The model under review builds one solid part; all positions refer to its coordinate system, in mm. A direction names the side the tool comes from. Coordinates: 2 decimals unless noted, no trailing zeros. One line per item, written item: value.
```python
from build123d import *

# Parameters (mm, degrees)
SKETCH3_R           = 3.512937447
SKETCH3_R_2         = 2.5
BOSS_EXTRUDE3_DEPTH = 13
CUT_EXTRUDE9_START  = -13.999999262
CUT_EXTRUDE9_DEPTH  = 13.999999262


# Read off the part's stored shape, not the designer's step: Cut-Extrude9
with BuildPart() as part:
    # Sketch1 → Revolve1 (revolve)
    with BuildSketch(Plane.XY, mode=Mode.PRIVATE) as revolve1_sk:
        with BuildLine():
            Line((-5.977318778, 9), (5.977318778, 9))
            add(Edge.make_bspline(
                [(5.977318778, 9), (5.971811367, 8.975222227), (5.562087836, 7.215033632), (4.069266539, 5.252557202), (1.935066771, 3.855081597), (0.019003444, 3.516133425), (0, 3.512937447)],
                knots=[0.019778015, 0.019778015, 0.019778015, 0.024722519, 0.375, 0.625, 0.982243258, 0.985794607, 0.985794607, 0.985794607], degree=2))
            Line((0, 3.512937447), (0, 2.5))
            add(Edge.make_bspline(
                [(6.999999581, 9.002422396), (5.87124706, 3.409561407), (0, 2.5)],
                knots=[0, 0, 0, 1, 1, 1], degree=2))
            Line((6.999999581, 9.002422396), (6.999999581, 11.002422396))
            Line((6.999999581, 11.002422396), (5.999999581, 11.002422396))
            Line((5.999999581, 11.002422396), (5.999999581, 10.9))
            ThreePointArc((5.999999581, 10.9), (5.736395684, 10.263603897), (5.099999581, 10))
            Line((5.099999581, 10), (-5.099999581, 10))
            ThreePointArc((-5.099999581, 10), (-5.736395684, 10.263603897), (-5.999999581, 10.9))
            Line((-5.999999581, 10.9), (-5.999999581, 11.002422396))
            Line((-5.999999581, 11.002422396), (-6.999999581, 11.002422396))
            Line((-6.999999581, 11.002422396), (-6.999999581, 9.002422396))
            Line((-6.999999581, 9.002422396), (-5.977318778, 9))
        make_face()
    revolve(revolve1_sk.sketch.rotate(Axis((0, 0, 0), (1, 0, 0)), 90), axis=Axis((0, 0, 0), (1, 0, 0)))

    # Sketch3 → Boss-Extrude3 (add)
    with BuildSketch(Plane.ZY.offset(6.999999581)):
        Circle(SKETCH3_R)
        Circle(SKETCH3_R_2, mode=Mode.SUBTRACT)
    extrude(amount=-BOSS_EXTRUDE3_DEPTH)

    # Cut-Extrude9 outline → Cut-Extrude9 (cut)
    with BuildSketch(Plane(origin=(6.999999581, 0, 0), x_dir=(0, 0, -1), z_dir=(1, 0, 0)).offset(CUT_EXTRUDE9_START)):
        with BuildLine():
            ThreePointArc((2.343182528, 2.617293478), (2.746525092, 2.190280673), (3.07307963, 1.702031461))
            Line((3.07307963, 1.702031461), (7.875221607, 4.361707651))
            ThreePointArc((7.875221607, 4.361707651), (7.038377248, 5.612918556), (6.004752201, 6.707202099))
            Line((6.004752201, 6.707202099), (2.343182528, 2.617293478))
        make_face()
        with BuildLine():
            ThreePointArc((3.50723285, -0.200118078), (3.424860771, -0.781702122), (3.24673559, -1.341431145))
            Line((3.24673559, -1.341431145), (8.320240718, -3.437615944))
            ThreePointArc((8.320240718, -3.437615944), (8.776712871, -2.003227439), (8.98780352, -0.512832208))
            Line((8.98780352, -0.512832208), (3.50723285, -0.200118078))
        make_face()
        with BuildLine():
            ThreePointArc((-0.585332029, 3.463829661), (0, 3.512937447), (0.585332029, 3.463829661))
            Line((0.585332029, 3.463829661), (1.5, 8.876576423))
            ThreePointArc((1.5, 8.876576423), (0, 9.002422396), (-1.5, 8.876576423))
            Line((-1.5, 8.876576423), (-0.585332029, 3.463829661))
        make_face()
        with BuildLine():
            ThreePointArc((2.030265301, -2.866836639), (1.524206435, -3.165047275), (0.975533429, -3.374768738))
            Line((0.975533429, -3.374768738), (2.499948867, -8.648344619))
            ThreePointArc((2.499948867, -8.648344619), (3.90600469, -8.110902314), (5.202855471, -7.346693402))
            Line((5.202855471, -7.346693402), (2.030265301, -2.866836639))
        make_face()
        with BuildLine():
            ThreePointArc((-3.07307963, 1.702031461), (-2.746525092, 2.190280673), (-2.343182528, 2.617293478))
            Line((-2.343182528, 2.617293478), (-6.004752201, 6.707202099))
            ThreePointArc((-6.004752201, 6.707202099), (-7.038377248, 5.612918556), (-7.875221607, 4.361707651))
            Line((-7.875221607, 4.361707651), (-3.07307963, 1.702031461))
        make_face()
        with BuildLine():
            ThreePointArc((-0.975533429, -3.374768738), (-1.524206435, -3.165047275), (-2.030265301, -2.866836639))
            Line((-2.030265301, -2.866836639), (-5.202855471, -7.346693402))
            ThreePointArc((-5.202855471, -7.346693402), (-3.90600469, -8.110902314), (-2.499948867, -8.648344619))
            Line((-2.499948867, -8.648344619), (-0.975533429, -3.374768738))
        make_face()
        with BuildLine():
            ThreePointArc((-3.24673559, -1.341431145), (-3.424860771, -0.781702122), (-3.50723285, -0.200118078))
            Line((-3.50723285, -0.200118078), (-8.98780352, -0.512832208))
            ThreePointArc((-8.98780352, -0.512832208), (-8.776712871, -2.003227439), (-8.320240718, -3.437615944))
            Line((-8.320240718, -3.437615944), (-3.24673559, -1.341431145))
        make_face()
    extrude(amount=CUT_EXTRUDE9_DEPTH, mode=Mode.SUBTRACT)


solid = part.part
```
(1) Tool access review of faces 1 (the flat face through (6, -2, 2)), 2 (the cylindrical face through (-0.1, 5.6, -7.05)), 3 (the cylindrical face through (0.084, 8.124, 3.873)): name each direction out of +Z, -Z, +X, -X, +Y, -Y from which nothing blocks a thin tool from reaching the whole face with its end or side.
Geometry results:
face 1: +X
face 2: +X, -X
face 3: -X
(2) We need section A-A, the plane z = 0. Count the separate pieces of the cut face and the enclosed holes in it, plus the area to 3 significant figures.
Geometry results:
separate pieces: 3
enclosed holes: 0
area: 66.6 mm2
(3) For L1, parallel to Z at x = -4.5, y = 1.5; L2, parallel to Y at x = 3, z = 1.5; L3, parallel to Y at x = 1.5, z = 1.5, list the stretches that pass through material, from the lowest coordinate up.
Geometry results:
L1: z = -9.89 to -8.87, -3.18 to -2, 2 to 3.18, 8.87 to 9.89
L2: y = -9.89 to -8.87, -3.18 to -2, 2 to 4.3, 8.87 to 9.89
L3: y = -9.89 to -8.87, -3.18 to -2, 2 to 3.58, 8.87 to 9.89
(4) Mouldability with a two-part tool opening along Y and no side actions: class faces 4 (the cylindrical face through (-6.507, -3.305, 10.494)), 5 (the cylindrical face through (0, -9, 0)) as +Y half, -Y half, draft (parallel to the pull), parting line (faces both ways), or undercut.
Geometry results:
face 4: parting line
face 5: undercut
(5) Insertion check: pin 1 Ø7.5 at (y, z) = (1, -0.5) entering from +X; pin 2 Ø10 at (y, z) = (-6, 6) entering from +X; pin 3 Ø5 at (x, y) = (2, -7.5) entering from +Z; pin 4 Ø11 at (y, z) = (-1, -1) entering from +X. Each pin has a flat end and moves straight along its axis. Give the tip position at first contact, or say it passes through.
Geometry results:
pin 1: stops at x = 6
pin 2: stops at x = 7
pin 3: stops at z = 8.66
pin 4: stops at x = 6.34
